Verification items for the finished model (mm, model axes). A direction names the side the tool comes from. Coordinates: 2 decimals unless noted, no trailing zeros. Order: outer loops, then holes, each group sorted by start corner. A loop starts at its lowest first (then second) coordinate and runs counter-clockwise, first axis right, second up. Notation, with made-up numbers: (26.5, 2) -> (55.5, 2) arc R12 cw to (55.5, 22) -> close; hole circle Ø8 at (23, 61.25). An arc over 180 degrees is marked (long way). Answer as CSV lines item,"result".
```python
from build123d import *

# Parameters (mm, degrees)
SKETCH019_R           = 22.86
PAD003_DEPTH          = 25.4
SKETCH021_R           = 1.55
POCKET017_DEPTH       = 164.33691
POLARPATTERN007_COUNT = 5
SKETCH022_W           = 45.72
SKETCH022_H           = 45.72
PAD004_DEPTH          = 10
SKETCH023_W           = 5.15
SKETCH023_H           = 5.8
POCKET018_DEPTH       = 45.721
SKETCH025_R           = 4.7
POCKET020_DEPTH       = 5.21
SKETCH028_R           = 6
POCKET023_DEPTH       = 35.401
SKETCH027_R           = 1.5
POCKET024_DEPTH       = 10
SKETCH029_R           = 4.7
POCKET025_DEPTH       = 5.21
SKETCH031_W           = 9.4
SKETCH031_H           = 3
POCKET027_DEPTH       = 35.401
SKETCH034_R           = 3.1645
POCKET029_DEPTH       = 45.721
SKETCH030_W           = 45.72
SKETCH030_H           = 45.72
POCKET030_DEPTH       = 10


with BuildPart() as part:
    # Sketch019 → Pad003 (new body)
    with BuildSketch(Plane.XY):
        Circle(SKETCH019_R)
    extrude(amount=PAD003_DEPTH)

    # Sketch021 → Pocket017 (cut, through all)
    with BuildSketch(Plane(origin=(0, 0, 0), x_dir=(1, 0, 0), z_dir=(0, 0, -1))):
        with Locations((0, 16)):
            Circle(SKETCH021_R)
    pocket017 = extrude(amount=-POCKET017_DEPTH, mode=Mode.SUBTRACT)

    # PolarPattern007: Pocket017 ×5 about axis
    polarpattern007_axis = Axis((0, 0, 0), (0, 0, -1))
    for i in range(1, POLARPATTERN007_COUNT):
        add(pocket017.rotate(polarpattern007_axis, i * 360 / POLARPATTERN007_COUNT), mode=Mode.SUBTRACT)

    # Sketch022 (on Face2 of PolarPattern007) → Pad004 (join)
    with BuildSketch(Plane(origin=(0, 0, 0), x_dir=(1, 0, 0), z_dir=(0, 0, -1))):
        Rectangle(SKETCH022_W, SKETCH022_H)
    extrude(amount=PAD004_DEPTH)

    # Sketch023 (on Face7 of Pad004) → Pocket018 (cut, through all)
    with BuildSketch(Plane(origin=(0, 22.86, 0), x_dir=(-1, 0, 0), z_dir=(0, 1, 0))):
        with Locations((0, 12.7)):
            Rectangle(SKETCH023_W, SKETCH023_H)
    extrude(amount=-POCKET018_DEPTH, mode=Mode.SUBTRACT)

    # Sketch025 → Pocket020 (cut)
    with BuildSketch(Plane.XZ.offset(22.86)):
        with Locations((0, 12.7)):
            Circle(SKETCH025_R)
    extrude(amount=-POCKET020_DEPTH, mode=Mode.SUBTRACT)

    # Sketch028 → Pocket023 (cut, through all)
    with BuildSketch(Plane.XY.offset(25.4)):
        Circle(SKETCH028_R)
    extrude(amount=-POCKET023_DEPTH, mode=Mode.SUBTRACT)

    # Sketch027 (on Face14 of Pocket023) → Pocket024 (cut)
    with BuildSketch(Plane(origin=(-22.86, 0, 0), x_dir=(0, -1, 0), z_dir=(-1, 0, 0))):
        with Locations((0, 12.7)):
            Circle(SKETCH027_R)
    extrude(amount=-POCKET024_DEPTH, mode=Mode.SUBTRACT)

    # Sketch029 (on Face19 of Pocket024) → Pocket025 (cut)
    with BuildSketch(Plane(origin=(0, 22.86, 0), x_dir=(-1, 0, 0), z_dir=(0, 1, 0))):
        with Locations((0, 12.7)):
            Circle(SKETCH029_R)
    extrude(amount=-POCKET025_DEPTH, mode=Mode.SUBTRACT)

    # Sketch031 → Pocket027 (cut, through all)
    with BuildSketch(Plane.XY.offset(25.4)):
        with Locations((0, 19.9)):
            Rectangle(SKETCH031_W, SKETCH031_H)
        with Locations((0, -19.9)):
            Rectangle(SKETCH031_W, SKETCH031_H)
    extrude(amount=-POCKET027_DEPTH, mode=Mode.SUBTRACT)

    # Sketch034 → Pocket029 (cut, through all)
    with BuildSketch(Plane.XZ.offset(22.86)):
        with Locations((0, 12.7)):
            Circle(SKETCH034_R)
    extrude(amount=-POCKET029_DEPTH, mode=Mode.SUBTRACT)

    # Sketch030 (on Face31 of Pocket029) → Pocket030 (cut)
    with BuildSketch(Plane(origin=(0, 0, -10), x_dir=(1, 0, 0), z_dir=(0, 0, -1))):
        Rectangle(SKETCH030_W, SKETCH030_H)
    extrude(amount=-POCKET030_DEPTH, mode=Mode.SUBTRACT)


solid = part.part
```
Item 1: Section check D-D, the plane x = 4. Count the separate pieces of the cut face and the enclosed holes in it, plus the area to 3 significant figures.
Answer list:
separate pieces,"6"
enclosed holes,"0"
area,"745 mm2"
Item 2: Release check for a two-part mould opening along Y. For faces 1 (the cylindrical face through (10.55, -20.28, 12.52)), 2 (the flat face through (-12.86, 0, 13)), 3 (the flat face through (-2, -11, 9.8)) record: +Y half, -Y half, draft (parallel to the pull), parting line (faces both ways), or undercut.
Answer list:
face 1,"parting line"
face 2,"undercut"
face 3,"draft"
Item 3: Section check B-B, the plane x = -9. Record the boundary of the cut face in (y, z).
Answer list:
outline,"(-21.01, 0) -> (11.45, 0) -> (11.45, 25.4) -> (-21.01, 25.4) -> close; (14.44, 0) -> (21.01, 0) -> (21.01, 25.4) -> (14.44, 25.4) -> close"
Item 4: Section check C-C, the plane y = 7. Record the boundary of the cut face in (x, z) (1 decimal), plus the area to 3 significant figures.
Answer list:
outline,"(-21.8, 0) -> (21.8, 0) -> (21.8, 25.4) -> (-21.8, 25.4) -> close; hole (-2.6, 9.8) -> (-1.3, 9.8) arc R3.2 ccw to (1.3, 9.8) -> (2.6, 9.8) -> (2.6, 10.9) arc R3.2 ccw to (2.6, 14.5) -> (2.6, 15.6) -> (1.3, 15.6) arc R3.2 ccw to (-1.3, 15.6) -> (-2.6, 15.6) -> (-2.6, 14.5) arc R3.2 ccw to (-2.6, 10.9) -> close"
area,"1,070 mm2"
Item 5: Tool access check on faces 4 (the cylindrical face through (-17.93, 0.325, 11.236)), 5 (the flat face through (2, -11, 15.6)), 6 (the flat face through (4.7, -20, 13)). Record the directions out of +Z, -Z, +X, -X, +Y, -Y that give a thin tool (end or side, any length) a straight path to the whole face; none if there is none.
Answer list:
face 4,"-X"
face 5,"+Y, -Y"
face 6,"+Z, -Z"
Item 6: Section check A-A, the plane y = 0. Record the boundary of the cut face in (x, z).
Answer list:
outline,"(-22.86, 0) -> (-6, 0) -> (-6, 25.4) -> (-22.86, 25.4) -> (-22.86, 14.2) -> (-12.86, 14.2) -> (-12.86, 11.2) -> (-22.86, 11.2) -> close; (6, 0) -> (22.86, 0) -> (22.86, 25.4) -> (6, 25.4) -> close"
Item 7: Thickness scan on line 1 (Y direction, x = 0, z = 20.5); line 2 (Z direction, x = 0, y = -21.95); line 3 (Y direction, x = 4, z = 2). Record the ranges inside material, lowest first.
Answer list:
line 1,"-22.86 to -21.4, -18.4 to -17.55, -14.45 to -6, 6 to 18.4, 21.4 to 22.86"
line 2,"0 to 8, 17.4 to 25.4"
line 3,"-22.51 to -21.4, -18.4 to -4.47, 4.47 to 18.4, 21.4 to 22.51"
Item 8: Depth check by flat-ended pin: pin 1 Ø0.9 at (y, z) = (19, 11) entering from +X; pin 2 Ø7.5 at (x, z) = (-1, 12.5) entering from +Y; pin 3 Ø1.2 at (y, z) = (-12, 15) entering from -X. Enter the tip coordinate at first touch or a pass-through.
Answer list:
pin 1,"x = 13.36"
pin 2,"y = 22.5"
pin 3,"x = -19.81"
